Source: three-view drawing plus pictorial views. Frame: mm from the lowest corner of the part. Coordinates: 2 decimals unless noted, no trailing zeros. Write each loop counter-clockwise with the first axis right and the second up, starting at its lowest first coordinate (ties: lowest second). Pieces come first, ordered by that corner, then holes. Notation, with made-up numbers: (-24, 75) - (7, 75) arc R7 ccw to (7, 81) - close; hole circle Ø10 at (-38, 47). An arc over 180 degrees is marked (long way). Answer as a JSON object with one key per item and string values. Group by question number.
Item 1: First-contact query: pin 1 Ø3 at (x, z) = (27, 4) entering from -Y; pin 2 Ø4.5 at (x, y) = (25, 25) entering from +Z. Flat tips, straight axial feed; report the tip coordinate or a pass-through.
Item 2: Line query: line 1 along Y through (x, z) = (25, 16.75); line 2 along Y through (x, z) = (25, 7); line 3 along X through (y, z) = (26, 4.5). Output: solid intervals per line, ascending. Write a range as from..to.
Item 3: Section A-A on x = 25. Return loops of the section in (y, z).
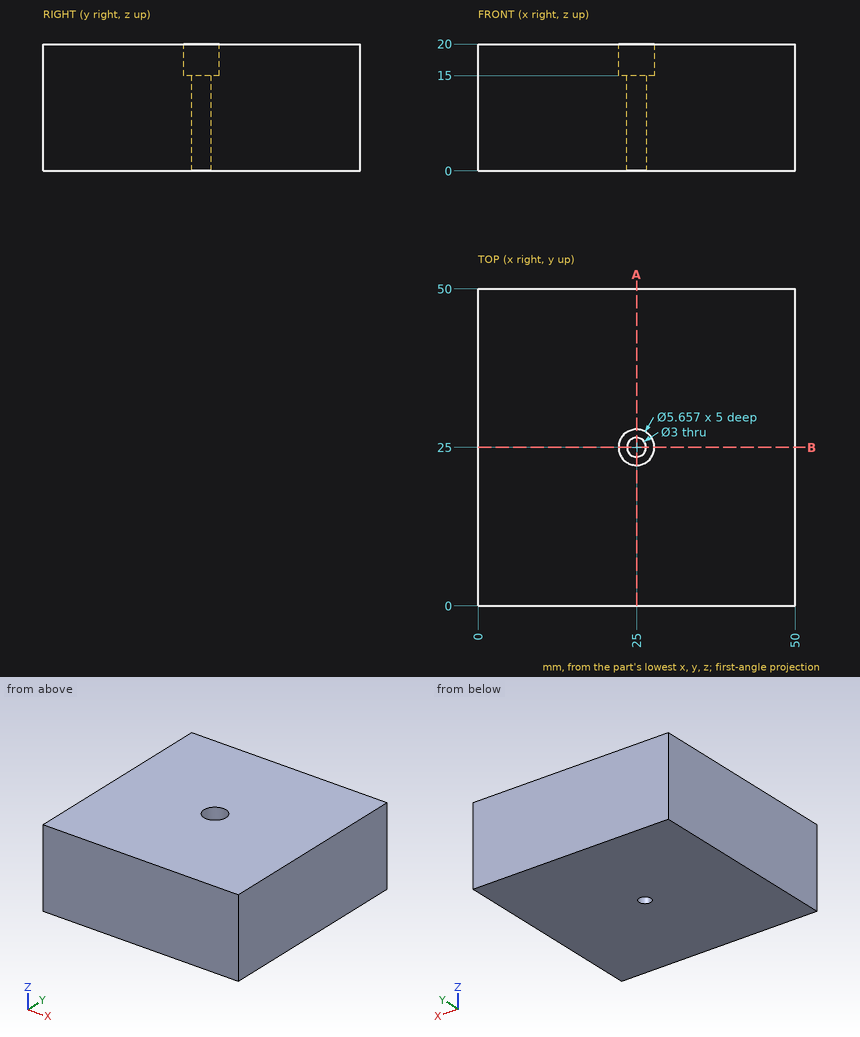
Checks:
{
 "1": {"pin 1": "y = 0", "pin 2": "z = 15"},
 "2": {"line 1": "0..22.17, 27.83..50", "line 2": "0..23.5, 26.5..50", "line 3": "0..23.88, 26.12..50"},
 "3": {"outline": "(0, 0) - (23.5, 0) - (23.5, 15) - (22.17, 15) - (22.17, 20) - (0, 20) - close; (26.5, 0) - (50, 0) - (50, 20) - (27.83, 20) - (27.83, 15) - (26.5, 15) - close"}
}
